Input: part model. Units: mm. Frame: model coordinates. Face numbers are marked on the shaded views. A direction names the side the tool comes from. Round coordinates to 2 decimals unless told otherwise and drop trailing zeros. Loops run counter-clockwise (first coordinate to the right, second up) from the corner with the lowest first, then second, coordinate; pieces in that order, holes last. Notation, with made-up numbers: M 63.5,-37 L 80.5,-37 A13 cw 80.5,-29 Z; hole C 41.5,-15 d3. An arc over 180 degrees is marked long. Put each result on its own line as item: value. Start each with the question number.
1) Section A-A on y = 0. Output: boundary loops of the cut face in (x, z), plus the area to 3 significant figures.
2) Pin query (flat end, axial travel): pin 1 (10 mm diameter, centred on x = -18, y = 12, fed in from +Z); pin 2 (8.5 mm diameter, centred on x = 5.5, z = 39, fed in from -Y); pin 3 (22.5 mm diameter, centred on x = -15, z = 22, fed in from +Y). Return the tip coordinate at first contact, or that it passes through.
3) Section B-B on z = 14.5. Output: boundary loops of the cut face in (x, y), plus the area to 3 significant figures.
4) Section C-C on x = 0. Output: boundary loops of the cut face in (y, z).
5) Draft query along X for the marked faces 1, 2 and 3. Return one class per face: +X half, -X half, draft (parallel to the pull), parting line (faces both ways), or undercut.
6) Reachability of the marked faces 4, 5 and 6 from +Z, -Z, +X, -X, +Y, -Y: full face, straight path, thin tool, end or side. Return the list, or none.
7) Line query: probe 1 along X at (y, z) = (-20, 42.5); probe 2 along Y at (x, z) = (-19, 32); probe 3 along Z at (x, y) = (0, -25.1). Output: solid intervals per line, ascending.
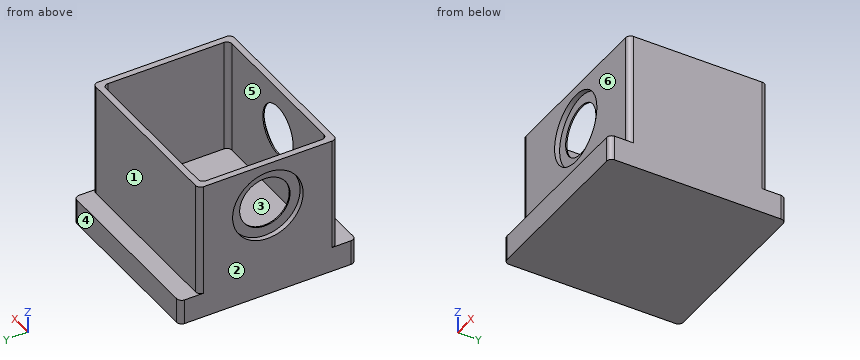
Autodesk Inventor part; units mm, degrees
ref_plane "YZ Plane" through (0, 0, 0) normal (1, 0, 0) x (0, 1, 0)
ref_plane "XZ Plane" through (0, 0, 0) normal (0, 1, 0) x (-1, 0, 0)
ref_plane "XY Plane" through (0, 0, 0) normal (0, 0, 1) x (1, 0, 0)
sketch "Sketch1" plane through (0, 0, 0) normal (0, 0, 1) x (1, 0, 0)
  line L0 (-33, 35) -> (33, 35)
  line L1 (35, 33) -> (35, -33)
  line L2 (33, -35) -> (-33, -35)
  line L3 (-35, -33) -> (-35, 33)
  arc A0 (-35, -33) -> (-33, -35) centre (-33, -33) ccw
  arc A1 (-33, 35) -> (-35, 33) centre (-33, 33) ccw
  arc A2 (35, 33) -> (33, 35) centre (33, 33) ccw
  arc A3 (33, -35) -> (35, -33) centre (33, -33) ccw
  point P0 (0, 0)
  point P1 (-35, 35)
  point P2 (35, -35)
  point P3 (35, 35)
  point P4 (-35, -35)
  dimension "d0" = 70
  dimension "d1" = 35
  dimension "d2" = 70
  dimension "d3" = 35
  dimension "d85" = 2
extrude "Extrusion1" add sketch "Sketch1" along normal blind 10
sketch "Sketch3" plane through (0, 0, 10) normal (0, 0, 1) x (1, 0, 0)
  line L0 (-33, 27.5) -> (33, 27.5)
  line L1 (35, 25.5) -> (35, -25.5)
  line L2 (33, -27.5) -> (-33, -27.5)
  line L3 (-35, -25.5) -> (-35, 25.5)
  line L4 (-35, 33) -> (-35, -33)
  line L5 (-30.5, 25) -> (30.5, 25)
  line L6 (32.5, 23) -> (32.5, -23)
  line L7 (30.5, -25) -> (-30.5, -25)
  line L8 (-32.5, -23) -> (-32.5, 23)
  arc A0 (-35, -25.5) -> (-33, -27.5) centre (-33, -25.5) ccw
  arc A1 (-32.5, -23) -> (-30.5, -25) centre (-30.5, -23) ccw
  arc A2 (33, -27.5) -> (35, -25.5) centre (33, -25.5) ccw
  arc A3 (30.5, -25) -> (32.5, -23) centre (30.5, -23) ccw
  arc A4 (32.5, 23) -> (30.5, 25) centre (30.5, 23) ccw
  arc A5 (-30.5, 25) -> (-32.5, 23) centre (-30.5, 23) ccw
  arc A6 (-33, 27.5) -> (-35, 25.5) centre (-33, 25.5) ccw
  arc A7 (35, 25.5) -> (33, 27.5) centre (33, 25.5) ccw
  point P0 (0, 0)
  point P1 (-35, 27.5)
  point P2 (35, -27.5)
  point P3 (35, 27.5)
  point P4 (-35, -27.5)
  point P5 (-35, 35)
  point P6 (-35, -35)
  point P7 (-32.5, 25)
  point P8 (32.5, -25)
  point P9 (32.5, 25)
  point P10 (-32.5, -25)
  dimension "d17" = 70
  dimension "d18" = 55
  dimension "d19" = 27.5
  dimension "d20" = 2.5
  dimension "d21" = 2.5
  dimension "d22" = 2.5
  dimension "d23" = 2.5
  dimension "d86" = 2
extrude "Extrusion2" add sketch "Sketch3" along normal blind 45
sketch "Sketch9" plane through (-35, -27.5, 10) normal (0, -1, 0) x (1, 0, 0)
  circle A0 centre (35, 27.5) radius 14
  line L0 (0, 0) -> (0, 45)
  line L1 (2, 0) -> (68, 0)
  point P0 (35, -10)
  point P1 (70, 0)
  dimension "d60" = 28
  dimension "d61" = 35
  dimension "d62" = 27.5
extrude "Extrusion8" cut sketch "Sketch9" against normal blind 2
sketch "Sketch10" plane through (0, -25.5, 37.5) normal (0, -1, 0) x (1, 0, 0)
  circle A0 centre (0, 0) radius 10
  point P0 (0, -37.5)
  dimension "d65" = 20
extrude "Extrusion9" cut sketch "Sketch10" against normal blind 2
sketch "Sketch13" plane through (-35, -35, 0) normal (-1, 0, 0) x (0, 0, 1)
  circle A0 centre (37.5, 35) radius 14
  line L0 (0, 68) -> (0, 2)
  line L1 (10, 68) -> (10, 60.5)
  point P0 (0, 35)
  point P1 (0, 35)
  point P2 (0, 0)
  point P3 (0, 70)
  point P4 (10, 70)
  point P5 (10, 62.5)
  point P6 (10, 7.5)
  dimension "d76" = 28
  dimension "d82" = 27.5
extrude "Extrusion12" cut sketch "Sketch13" against normal blind 2
sketch "Sketch14" plane through (-33, 0, 37.5) normal (-1, 0, 0) x (0, 0, 1)
  circle A0 centre (0, 0) radius 10
  line L0 (-37.5, 33) -> (-37.5, -33)
  line L1 (-27.5, 33) -> (-27.5, 25.5)
  point P0 (-37.5, 0)
  point P1 (-37.5, 0)
  point P2 (-37.5, -35)
  point P3 (-37.5, 35)
  point P4 (-27.5, 35)
  point P5 (-27.5, 27.5)
  point P6 (-27.5, -27.5)
  dimension "d80" = 20
  dimension "d81" = 27.5
extrude "Extrusion13" cut sketch "Sketch14" against normal blind 2
equation "\"d21\" = d20"
properties part number "sampleChamber_singlePiece_filipeSample"
Geometry results:
1. outline: M -35,0 L 35,0 L 35,55 L 32.5,55 L 32.5,10 L -32.5,10 L -32.5,27.5 L -33,27.5 L -33,23.5 L -35,23.5 Z; M -35,51.5 L -33,51.5 L -33,47.5 L -32.5,47.5 L -32.5,55 L -35,55 Z
1. area: 859 mm²
2. pin 1: stops at z = 10
2. pin 2: stops at y = 25
2. pin 3: stops at y = 27.5
3. outline: M -35,-25.5 A2 ccw -33,-27.5 L 33,-27.5 A2 ccw 35,-25.5 L 35,25.5 A2 ccw 33,27.5 L -33,27.5 A2 ccw -35,25.5 Z; hole M -32.5,-23 A2 ccw -30.5,-25 L 30.5,-25 A2 ccw 32.5,-23 L 32.5,23 A2 ccw 30.5,25 L -30.5,25 A2 ccw -32.5,23 Z
3. area: 600 mm²
4. outline: M -35,0 L 35,0 L 35,10 L 27.5,10 L 27.5,55 L 25,55 L 25,10 L -25,10 L -25,27.5 L -25.5,27.5 L -25.5,23.5 L -27.5,23.5 L -27.5,10 L -35,10 Z; M -27.5,51.5 L -25.5,51.5 L -25.5,47.5 L -25,47.5 L -25,55 L -27.5,55 Z
5. face 1: draft
5. face 2: -X half
5. face 3: undercut
6. face 4: +Z, -Z, +X, -X, +Y
6. face 5: +Z
6. face 6: +Z, +X, -X, -Y
7. probe 1: x = -35 to -32.5, 32.5 to 35
7. probe 2: y = -27.5 to -25, 25 to 27.5
7. probe 3: z = 0 to 27.5, 47.5 to 55
